Input: dimensioned drawing with shaded views. Units: mm. Origin: part minimum x, y, z. A direction names the side the tool comes from. Round coordinates to 2 decimals unless told otherwise and drop trailing zeros. Loops run counter-clockwise (first coordinate to the right, second up) from the corner with the lowest first, then second, coordinate; pieces in that order, holes last. Notation, with made-up numbers: (33.25, 52) - (39.25, 52) arc R14 ccw to (39.25, 73) - close; hole circle Ø5 at (71.5, 30.5). An arc over 180 degrees is marked (long way). Write each question's results on one line, items separated by ' | '.
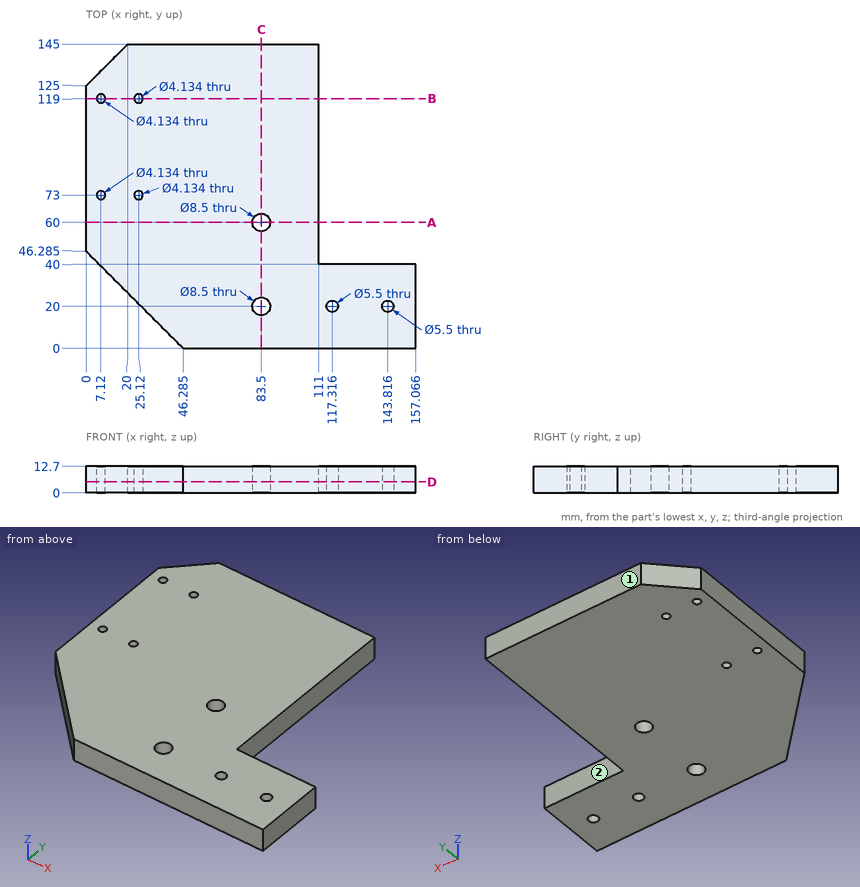
1. Section query C-C, the plane x = 83.5. Output: boundary loops of the cut face in (y, z), plus the area to 3 significant figures.
Answer:
outline: (0, 0) - (15.75, 0) - (15.75, 12.7) - (0, 12.7) - close; (24.25, 0) - (55.75, 0) - (55.75, 12.7) - (24.25, 12.7) - close; (64.25, 0) - (145, 0) - (145, 12.7) - (64.25, 12.7) - close | area: 1,630 mm^2
2. Section query D-D, the plane z = 5.25. Count the separate pieces of the cut face and the enclosed holes in it, plus the area to 3 significant figures.
Answer:
separate pieces: 1 | enclosed holes: 8 | area: 16,500 mm^2
3. Section query A-A, the plane y = 60. Output: boundary loops of the cut face in (x, z).
Answer:
outline: (0, 0) - (79.25, 0) - (79.25, 12.7) - (0, 12.7) - close; (87.75, 0) - (111, 0) - (111, 12.7) - (87.75, 12.7) - close
4. Section query B-B, the plane y = 119. Output: boundary loops of the cut face in (x, z), plus the area to 3 significant figures.
Answer:
outline: (0, 0) - (5.05, 0) - (5.05, 12.7) - (0, 12.7) - close; (9.19, 0) - (23.05, 0) - (23.05, 12.7) - (9.19, 12.7) - close; (27.19, 0) - (111, 0) - (111, 12.7) - (27.19, 12.7) - close | area: 1,300 mm^2
5. Set-up query: the marked faces 1 and 2. Return all of +Z, -Z, +X, -X, +Y, -Y with unobstructed straight access to the full face (end or side cutting, diameter ignored); none if empty.
Answer:
face 1: +Z, -Z, +X, -X, +Y | face 2: +Z, -Z, +X, +Y
6. Line query: line 1 (Y direction, x = 83.5, z = 8.25); line 2 (X direction, y = 119, z = 8.25); line 3 (X direction, y = 60, z = 9.25). Output: solid intervals per line, ascending. Write a range as [from, to].
Answer:
line 1: [0, 15.75], [24.25, 55.75], [64.25, 145] | line 2: [0, 5.05], [9.19, 23.05], [27.19, 111] | line 3: [0, 79.25], [87.75, 111]
7. Contact query for a flat-ended pin moving along its axis: pin 1 (1 mm diameter, centred on y = 63, z = 5.5, fed in from +X). Output: stop coordinate, or through.
Answer:
pin 1: x = 111
